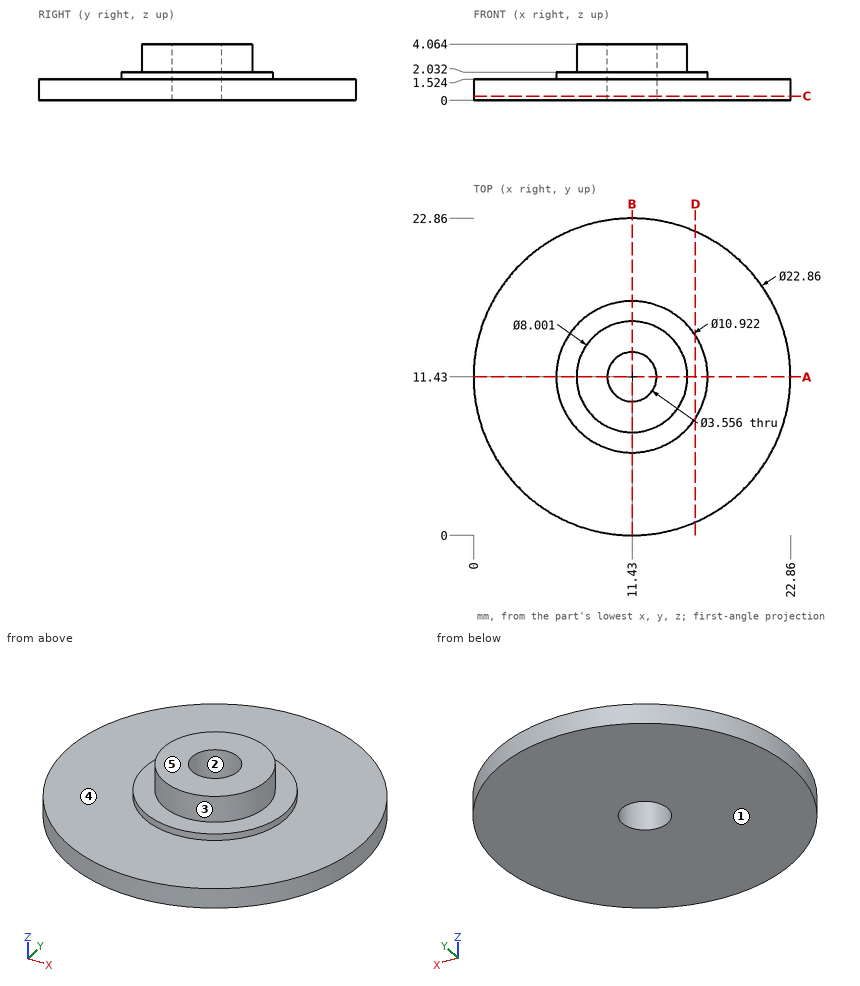
Check sheet for the drawn part. Datum: minimum x, y, z corner. Units: mm. A direction names the side the tool comes from. Round coordinates to 2 decimals unless told otherwise and drop trailing zeros. Order: outer loops, then holes, each group sorted by start corner. A loop starts at its lowest first (then second) coordinate and runs counter-clockwise, first axis right, second up.
1) Section check D-D (x = 16). Record the boundary of the cut face in (y, z), and give its area (3 significant figures).
2) Mould release check, pull along X, two halves, no side actions. Record for the marked faces 1, 2 and 3: +X half, -X half, draft (parallel to the pull), parting line (faces both ways), or undercut.
3) Section check C-C (z = 0.3). Record the boundary of the cut face in (x, y), and give its area (3 significant figures).
4) Section check A-A (y = 11.43). Record the boundary of the cut face in (x, z).
5) Go/stop test with flat-tipped pins: pin 1 Ø1.5 at (x, z) = (4.5, 1.5) entering from -Y; pin 2 Ø2 at (x, z) = (15, 0.5) entering from -Y; pin 3 Ø3 at (x, y) = (11.43, 11.43) entering from -Z. Record where each tip stops, or that it passes through.
6) Scan lines: line 1 (Y direction, x = 11.5, z = 2.4); line 2 (Y direction, x = 11.43, z = 1.4); line 3 (Z direction, x = 17.5, y = 2.75). Record each from-to range of solid material in increasing order.
7) Tool access check on the marked faces 4 and 5. Record the directions out of +Z, -Z, +X, -X, +Y, -Y that give a thin tool (end or side, any length) a straight path to the whole face; none if there is none.
Result:
1. outline: (0.95, 0) - (21.91, 0) - (21.91, 1.52) - (14.42, 1.52) - (14.42, 2.03) - (8.44, 2.03) - (8.44, 1.52) - (0.95, 1.52) - close
1. area: 35.0 mm2
2. face 1: draft
2. face 2: undercut
2. face 3: parting line
3. outline: circle Ø22.86 at (11.43, 11.43); hole circle Ø3.56 at (11.43, 11.43)
3. area: 401 mm2
4. outline: (0, 0) - (9.65, 0) - (9.65, 4.06) - (7.43, 4.06) - (7.43, 2.03) - (5.97, 2.03) - (5.97, 1.52) - (0, 1.52) - close; (13.21, 0) - (22.86, 0) - (22.86, 1.52) - (16.89, 1.52) - (16.89, 2.03) - (15.43, 2.03) - (15.43, 4.06) - (13.21, 4.06) - close
5. pin 1: stops at y = 1.81
5. pin 2: stops at y = 0.29
5. pin 3: passes through
6. line 1: y = 7.43 to 9.65, 13.21 to 15.43
6. line 2: y = 0 to 9.65, 13.21 to 22.86
6. line 3: z = 0 to 1.52
7. face 4: +Z
7. face 5: +Z, +X, -X, +Y, -Y
